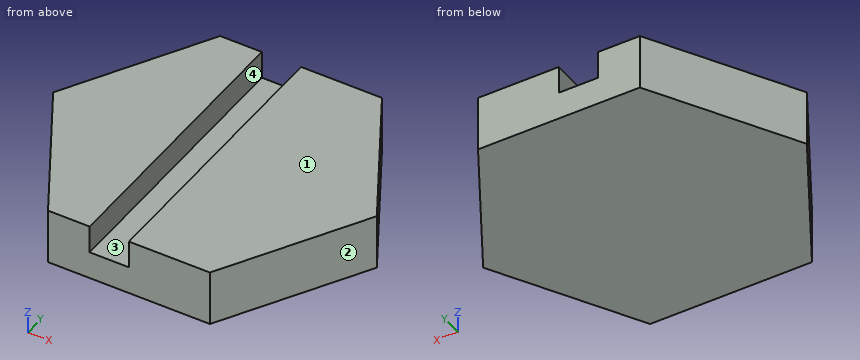
from build123d import *

# Parameters (mm, degrees)
SKETCH001_W           = 7
SKETCH001_H           = 60
EXTRUDE001_DEPTH      = 1
EXTRUDE001_DEPTH_BACK = 5
EXTRUDE_DEPTH         = 10


with BuildPart() as extrude001:
    # Sketch001 (on Face8 of Extrude) → Extrude001 (new body, two sides)
    with BuildSketch(Plane.XY.offset(10)) as extrude001_sk:
        with Locations((-3.5, 0)):
            Rectangle(SKETCH001_W, SKETCH001_H)
    extrude(amount=EXTRUDE001_DEPTH)
    extrude(extrude001_sk.sketch, amount=-EXTRUDE001_DEPTH_BACK)


with BuildPart() as cut:
    # Sketch → Extrude (new body)
    with BuildSketch(Plane.XY):
        Polygon((28.867513, 0), (14.433757, 25), (-14.433757, 25), (-28.867513, 0), (-14.433757, -25), (14.433757, -25), align=None)
    extrude(amount=EXTRUDE_DEPTH)

    # Cut: cut Extrude001
    add(extrude001.part, mode=Mode.SUBTRACT)


solid = cut.part
Source: CAD feature listing. Evaluate the final solid. Frame: model axes, mm. Face numbers are marked on the shaded views. Give positions to 0.01 mm unless a question says otherwise; leave off trailing zeros. Write each loop counter-clockwise with the first axis right and the second up, starting at its lowest first coordinate (ties: lowest second). Pieces come first, ordered by that corner, then holes. Notation, with made-up numbers: (84, -34.75) -> (92, -34.75) arc R28 ccw to (92, 3.25) -> close; hole circle Ø11 at (41, -4.75). An arc over 180 degrees is marked (long way). Return JSON: item names as keys, results as strings. Group by question number.
1. Section B-B, the plane y = 17. Output: boundary loops of the cut face in (x, z).
2. Section C-C, the plane z = 4. Output: boundary loops of the cut face in (x, y), then the cut area to 3 significant figures.
3. Mould query, pull axis X, two halves, no side actions, for the marked faces 1, 2, 3 and 4. Classes: +X half, -X half, draft (parallel to the pull), parting line (faces both ways), or undercut.
4. Section D-D, the plane x = -21.5. Output: boundary loops of the cut face in (y, z).
5. Section A-A, the plane z = 7.25. Output: boundary loops of the cut face in (x, y).
6. Material intervals for line 1 (Z direction, x = -6, y = 11); line 2 (X direction, y = -11, z = 4.25); line 3 (X direction, y = 16.5, z = 6.5), sorted ascending. Write a range as from..to.
7. Pin query (flat end, axial travel): pin 1 Ø2.5 at (y, z) = (5, 8.5) entering from -X; pin 2 Ø5.5 at (y, z) = (-8.5, 7.5) entering from +X; pin 3 Ø4 at (y, z) = (8.5, 3) entering from +X. Return the tip coordinate at first contact, or that it passes through.
Determined:
{
 "1": {"outline": "(-19.05, 0) -> (19.05, 0) -> (19.05, 10) -> (0, 10) -> (0, 5) -> (-7, 5) -> (-7, 10) -> (-19.05, 10) -> close"},
 "2": {"outline": "(-28.87, 0) -> (-14.43, -25) -> (14.43, -25) -> (28.87, 0) -> (14.43, 25) -> (-14.43, 25) -> close", "area": "2,170 mm2"},
 "3": {"face 1": "draft", "face 2": "+X half", "face 3": "undercut", "face 4": "undercut"},
 "4": {"outline": "(-12.76, 0) -> (12.76, 0) -> (12.76, 10) -> (-12.76, 10) -> close"},
 "5": {"outline": "(-28.87, 0) -> (-14.43, -25) -> (-7, -25) -> (-7, 25) -> (-14.43, 25) -> close; (0, -25) -> (14.43, -25) -> (28.87, 0) -> (14.43, 25) -> (0, 25) -> close"},
 "6": {"line 1": "z = 0..5", "line 2": "x = -22.52..22.52", "line 3": "x = -19.34..-7, 0..19.34"},
 "7": {"pin 1": "stops at x = -26.7", "pin 2": "stops at x = 25.55", "pin 3": "stops at x = 25.11"}
}
